from build123d import *

# Parameters (mm, degrees)
SKETCH1_R           = 4.5
SKETCH1_R_2         = 6.5
SKETCH1_R_3         = 1.75
BOSS_EXTRUDE1_DEPTH = 4
SKETCH2_R           = 2
CUT_EXTRUDE1_DEPTH  = 4
SKETCH3_R           = 2
CUT_EXTRUDE2_DEPTH  = 10
CUT_EXTRUDE3_START  = -10
CUT_EXTRUDE3_DEPTH  = 10


with BuildPart() as part:
    # Sketch1 → Boss-Extrude1 (new body)
    with BuildSketch(Plane(origin=(0, 0, 0), x_dir=(1, 0, 0), z_dir=(0, 1, 0))):
        with BuildLine():
            Line((-270, -14.5), (0, -14.5))
            Line((0, -14.5), (0, 340))
            Line((0, 340), (-175.463800793, 340))
            ThreePointArc((-175.463800793, 340), (-185.71684912, 335.753048327), (-189.963800793, 325.5))
            Line((-189.963800793, 325.5), (-189.963800793, 225.606590828))
            ThreePointArc((-189.963800793, 225.606590828), (-204.963800793, 210.606590828), (-189.963800793, 195.606590828))
            Line((-189.963800793, 195.606590828), (-189.963800793, 54.5))
            Line((-189.963800793, 54.5), (-229.963800793, 14.5))
            Line((-229.963800793, 14.5), (-270, 14.5))
            ThreePointArc((-270, 14.5), (-284.5, 0), (-270, -14.5))
        make_face()
        with Locations(Location((-270, 0, 0), (0, 0, 270))):
            Circle(SKETCH1_R, mode=Mode.SUBTRACT)
        with Locations(Location((-175.463800793, 325.5, 0), (0, 0, 270))):
            Circle(SKETCH1_R, mode=Mode.SUBTRACT)
        with Locations(Location((-189.963800793, 210.606590828, 0), (0, 0, 270))):
            Circle(SKETCH1_R_2, mode=Mode.SUBTRACT)
        with Locations(Location((-180.213800793, 210.606590828, 0), (0, 0, 270))):
            Circle(SKETCH1_R_3, mode=Mode.SUBTRACT)
        with Locations(Location((-189.963800793, 220.406590828, 0), (0, 0, 270))):
            Circle(SKETCH1_R_3, mode=Mode.SUBTRACT)
        with Locations(Location((-189.963800793, 200.806590828, 0), (0, 0, 270))):
            Circle(SKETCH1_R_3, mode=Mode.SUBTRACT)
        with Locations(Location((-199.713800793, 210.606590828, 0), (0, 0, 270))):
            Circle(SKETCH1_R_3, mode=Mode.SUBTRACT)
    boss_extrude1 = extrude(amount=BOSS_EXTRUDE1_DEPTH)

    # Mirror1: Boss-Extrude1 across plane
    add(boss_extrude1.mirror(Plane(origin=(0, 4, -340), x_dir=(0, 0, 1), z_dir=(-1, 0, 0))))

    # Sketch2 → Cut-Extrude1 (cut)
    with BuildSketch(Plane(origin=(0, 4, 0), x_dir=(1, 0, 0), z_dir=(0, 1, 0))):
        with Locations(Location((0, 305.5, 0), (0, 0, 270))):
            Circle(SKETCH2_R)
    extrude(amount=-CUT_EXTRUDE1_DEPTH, mode=Mode.SUBTRACT)

    # Sketch3 → Cut-Extrude2 (cut)
    with BuildSketch(Plane(origin=(0, 4, 0), x_dir=(1, 0, 0), z_dir=(0, 1, 0))):
        with Locations(Location((-170, 15.5, 0), (0, 0, 270))):
            Circle(SKETCH3_R)
        with Locations(Location((170, 15.5, 0), (0, 0, 270))):
            Circle(SKETCH3_R)
    extrude(amount=-CUT_EXTRUDE2_DEPTH, mode=Mode.SUBTRACT)

    # Sketch4 → Cut-Extrude3 (cut)
    with BuildSketch(Plane(origin=(0, 4, 0), x_dir=(1, 0, 0), z_dir=(0, 1, 0)).offset(CUT_EXTRUDE3_START)):
        with BuildLine():
            Line((-175.463800793, 311), (175.463800793, 311))
            ThreePointArc((175.463800793, 311), (185.71684912, 315.246951673), (189.963800793, 325.5))
            Line((189.963800793, 325.5), (382.257646385, 325.5))
            Line((382.257646385, 325.5), (382.257646385, -89.216188956))
            Line((382.257646385, -89.216188956), (-350.501872642, -89.216188956))
            Line((-350.501872642, -89.216188956), (-350.501872642, 325.5))
            Line((-350.501872642, 325.5), (-189.963800793, 325.5))
            ThreePointArc((-189.963800793, 325.5), (-185.71684912, 315.246951673), (-175.463800793, 311))
        make_face()
    extrude(amount=CUT_EXTRUDE3_DEPTH, mode=Mode.SUBTRACT)


solid = part.part
Check sheet for the modelled part. Datum: model origin and axes. Units: mm. Round coordinates to 2 decimals unless told otherwise and drop trailing zeros. Order: outer loops, then holes, each group sorted by start corner. A loop starts at its lowest first (then second) coordinate and runs counter-clockwise, first axis right, second up. Notation, with made-up numbers: M -24.75,-6 L -4.75,-6 A20 cw -4.75,22 Z; hole C 2,-17.75 d7. An arc over 180 degrees is marked long. One line per item, written item: value. Start each with the question number.
1. Scan lines: line 1 along X through (y, z) = (2.1, -325.5); line 2 along X through (y, z) = (3.25, -323.75); line 3 along Z through (x, y) = (173, 2.95). Record each from-to range of solid material in increasing order.
2. Gauge pin test, flat end, axial feed: P1, Ø2, axis at y = 2, z = -319, coming from the +X side. Record the tip position at first contact, or that the pin passes through.
3. Release check for a two-part mould opening along X. For faces 1 (the flat face through (3, 0, -326)), 2 (the cylindrical face through (174.11, 1.97, -321.21)) record: released by +X, released by -X, zero draft, split by the parting line, or undercut.
4. Section check A-A on y = 1.9. Enter the section's corners in (x, z), and give its area (3 significant figures).
Results found:
1. line 1: -189.96 to -179.96, -170.96 to 170.96, 179.96 to 189.96
1. line 2: -189.86 to -179.61, -171.32 to 171.32, 179.61 to 189.86
1. line 3: -340 to -329.27, -321.73 to -311
2. P1: x = 188.88
3. face 1: zero draft
3. face 2: undercut
4. outline: M -175.46,-340 L 175.46,-340 A14.5 ccw 175.46,-311 L -175.46,-311 A14.5 ccw Z; hole C -175.46,-325.5 d9; hole C 175.46,-325.5 d9
4. area: 10,700 mm^2
